Check sheet for the modelled part. Datum: model origin and axes. Units: mm. A direction names the side the tool comes from. Round coordinates to 2 decimals unless told otherwise and drop trailing zeros. Order: outer loops, then holes, each group sorted by start corner. A loop starts at its lowest first (then second) coordinate and runs counter-clockwise, first axis right, second up.
Q1. Cross-section at A-A on x = 57. Record the cut outline in (y, z), then the cut area to 3 significant figures.
Q2. Cross-section at C-C on y = -56.5. Record the cut outline in (x, z), then the cut area to 3 significant figures.
Q3. Depth check by flat-ended pin: P1, Ø3, axis at x = 36.5, y = -104.5, coming from the +Z side; P2, Ø1.5, axis at x = 67, z = -3, coming from the -Y side; P3, Ø14, axis at x = 84.5, z = 3.5, coming from the -Y side; P4, Ø5, axis at y = -40, z = 28.5, coming from the -X side. Enter the tip coordinate at first touch or a pass-through.
Q4. Mould release check, pull along Y, two halves, no side actions. Record for faces 1 (the flat face through (37.57, -0.05, 42.32)), 2 (the flat face through (25.4, -81, 1)), 3 (the flat face through (82, 0, -16.387)): +Y half, -Y half, draft (parallel to the pull), parting line (faces both ways), or undercut.
Q5. Set-up check for faces 4 (the flat face through (82, -23.097, 0)), 5 (the flat face through (82, 23.097, 0)), 6 (the flat face through (82, 0, 16.387)): record each of +Z, -Z, +X, -X, +Y, -Y from which the full face is reachable in a straight line by a thin tool's end or side.
Q6. Scan lines: probe 1 along Y at (x, z) = (61, 4); probe 2 along Y at (x, z) = (27, -11); probe 3 along X at (y, z) = (-27.5, -0.5). Record each from-to range of solid material in increasing order.
Q7. Cross-section at D-D on z = 10. Record the cut outline in (x, y), then the cut area to 3 significant figures.
Q8. Cross-section at B-B on x = 12. Record the cut outline in (y, z).
from build123d import *

# Parameters (mm, degrees)
F1_DEPTH = 76.2
F2_R     = 38.089207
F2_R_2   = 16.306918
F3_DEPTH = 50.8
F4_W     = 46.19369
F4_H     = 32.77332
F5_DEPTH = 12.7


with BuildPart() as f1:
    # F0 (on Right) → F1 (new body)
    with BuildSketch(Plane.YZ):
        with BuildLine():
            ThreePointArc((-61.721072, -60.821969), (-29.022062, -37.905089), (-16.467663, 0))
            ThreePointArc((-16.467663, 0), (-29.022062, 37.905089), (-61.721072, 60.821969))
            ThreePointArc((-61.721072, 60.821969), (-143.467663, 0), (-61.721072, -60.821969))
        make_face()
        with BuildLine():
            ThreePointArc((-61.721072, 60.821969), (-29.022062, 37.905089), (-16.467663, 0))
            ThreePointArc((-16.467663, 0), (-29.022062, -37.905089), (-61.721072, -60.821969))
            Line((-61.721072, -60.821969), (59.922866, -24.328788))
            ThreePointArc((59.922866, -24.328788), (27.22423, 0), (59.922866, 24.328788))
            Line((59.922866, 24.328788), (-61.721072, 60.821969))
        make_face()
        with BuildLine():
            ThreePointArc((78.02423, 0), (73.00247, 15.162035), (59.922866, 24.328788))
            ThreePointArc((59.922866, 24.328788), (27.22423, 0), (59.922866, -24.328788))
            ThreePointArc((59.922866, -24.328788), (73.00247, -15.162035), (78.02423, 0))
        make_face()
    extrude(amount=F1_DEPTH)

    # F2 (on face) → F3 (cut)
    with BuildSketch(Plane.YZ.offset(76.2)):
        with Locations((-79.967663, 0)):
            Circle(F2_R)
        with Locations((52.62423, 0)):
            Circle(F2_R_2)
    extrude(amount=-F3_DEPTH, mode=Mode.SUBTRACT)

    # F4 (on face) → F5 (join)
    with BuildSketch(Plane.YZ.offset(76.2)):
        Rectangle(F4_W, F4_H)
    extrude(amount=F5_DEPTH)


solid = f1.part
Results found:
1. outline: (-61.72, -60.82) - (59.92, -24.33) arc R25.4 ccw to (78.02, 0) arc R25.4 ccw to (59.92, 24.33) - (-61.72, 60.82) arc R63.5 ccw (long way) to start; hole circle Ø76.18 at (-79.97, 0); hole circle Ø32.61 at (52.62, 0)
1. area: 14,200 mm2
2. outline: (0, -59.26) - (76.2, -59.26) - (76.2, -30) - (25.4, -30) - (25.4, 30) - (76.2, 30) - (76.2, 59.26) - (0, 59.26) - close
2. area: 5,980 mm2
3. P1: stops at z = 59.18
3. P2: stops at y = -143.43
3. P3: stops at y = -23.1
3. P4: stops at x = 0
4. face 1: +Y half
4. face 2: undercut
4. face 3: draft
5. face 4: +Z, -Z, +X, -Y
5. face 5: +Z, -Z, +X, +Y
5. face 6: +Z, +X, +Y, -Y
6. probe 1: y = -143.34 to -117.85, -42.09 to 36.82, 68.43 to 77.71
6. probe 2: y = -142.51 to -116.43, -43.5 to 40.59, 64.66 to 75.52
6. probe 3: x = 0 to 76.2
7. outline: (0, -142.68) - (76.2, -142.68) - (76.2, -116.72) - (25.4, -116.72) - (25.4, -43.21) - (76.2, -43.21) - (76.2, -23.1) - (88.9, -23.1) - (88.9, 23.1) - (76.2, 23.1) - (76.2, 39.74) - (25.4, 39.74) - (25.4, 65.51) - (76.2, 65.51) - (76.2, 75.97) - (0, 75.97) - close
7. area: 12,200 mm2
8. outline: (-61.72, -60.82) - (59.92, -24.33) arc R25.4 ccw to (78.02, 0) arc R25.4 ccw to (59.92, 24.33) - (-61.72, 60.82) arc R63.5 ccw (long way) to start
